Geometry check sheet. Reference: the model listing, model coordinates, mm. Face numbers are marked on the shaded views. A direction names the side the tool comes from. Give positions to 0.01 mm unless a question says otherwise; leave off trailing zeros. Order: outer loops, then holes, each group sorted by start corner. A loop starts at its lowest first (then second) coordinate and runs counter-clockwise, first axis right, second up. Notation, with made-up numbers: M 35.25,16 L 68.25,16 A31 ccw 68.25,52 Z; hole C 51,57 d10. An arc over 180 degrees is marked long. Use CSV: the item, a comma, the result in double quotes. Start each with the question number.
from build123d import *

# Parameters (mm, degrees)
F0_W     = 3.5
F0_H     = 4.8
F1_DEPTH = 19
F3_D     = 5
F3_DEPTH = 10
F3_TIP   = 1.5021515476


with BuildPart() as f1:
    # F0 (on Right) → F1 (new body)
    with BuildSketch(Plane.YZ):
        with Locations((-19.75, 3.4)):
            Rectangle(F0_W, F0_H)
        Polygon((21.5, -1), (21.5, 1), (18, 1), (-18, 1), (-21.5, 1), (-21.5, -1), align=None)
        with Locations((19.75, 3.4)):
            Rectangle(F0_W, F0_H)
    extrude(amount=F1_DEPTH)

    # F3
    with Locations(Plane(origin=(0, 0, -1), x_dir=(1, 0, 0), z_dir=(0, 0, -1))):
        with Locations((9.5, 14), (9.5, -14)):
            Hole(F3_D / 2, depth=F3_DEPTH)
            with Locations((0, 0, -(F3_DEPTH + F3_TIP / 2))):  # 118° drill point
                Cone(0, F3_D / 2, F3_TIP, mode=Mode.SUBTRACT)


solid = f1.part
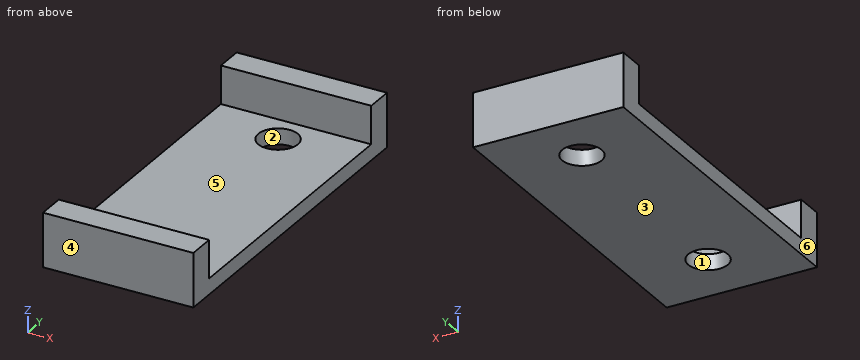
(1) Draft check along Y on the marked faces 1, 2, 3 and 4. Enter one of: +Y half, -Y half, draft (parallel to the pull), parting line (faces both ways), or undercut.
(2) Access from +Z, -Z, +X, -X, +Y, -Y to the whole of each face (thin tool, end or side, straight path). Record for the marked faces 5 and 6.
(3) Thickness scan on line 1 (Y direction, x = 9.5, z = -0.1); line 2 (Y direction, x = 4.5, z = 4.25); line 3 (Y direction, x = 7.5, z = 0). Record the ranges inside material, lowest first.
(4) Sectioned sample at C-C on z = 2.75. Record the cut outline in (x, y), then the cut area to 3 significant figures.
(5) Sectioned sample at B-B on x = 7.5. Record the cut outline in (y, z), then the cut area to 3 significant figures.
(6) Go/stop test with flat-tipped pins: P1, Ø5.5, axis at x = 12.5, y = 5.5, coming from the +Z side; P2, Ø4, axis at x = 9.5, y = -14, coming from the +Z side. Record where each tip stops, or that it passes through.
(7) Sectioned sample at D-D on x = 3.5. Record the cut outline in (y, z).
(8) Sectioned sample at A-A on y = 16. Record the cut outline in (x, z), then the cut area to 3 significant figures.
Responses:
1,face 1,"undercut"
1,face 2,"undercut"
1,face 3,"draft"
1,face 4,"-Y half"
2,face 5,"+Z, +X, -X"
2,face 6,"+Z, -Z, -X, +Y, -Y"
3,line 1,"-21.5 to -16.5, -11.5 to 11.5, 16.5 to 21.5"
3,line 2,"-21.5 to -18, 18 to 21.5"
3,line 3,"-21.5 to -15.5, -12.5 to 12.5, 15.5 to 21.5"
4,outline,"M 0,-21.5 L 19,-21.5 L 19,-18 L 0,-18 Z; M 0,18 L 19,18 L 19,21.5 L 0,21.5 Z"
4,area,"133 mm2"
5,outline,"M -21.5,-1 L -15.5,-1 L -15.5,1 L -18,1 L -18,5.8 L -21.5,5.8 Z; M -12.5,-1 L 12.5,-1 L 12.5,1 L -12.5,1 Z; M 15.5,-1 L 21.5,-1 L 21.5,5.8 L 18,5.8 L 18,1 L 15.5,1 Z"
5,area,"108 mm2"
6,P1,"z = 1"
6,P2,"through"
7,outline,"M -21.5,-1 L 21.5,-1 L 21.5,5.8 L 18,5.8 L 18,1 L -18,1 L -18,5.8 L -21.5,5.8 Z"
8,outline,"M 0,-1 L 8,-1 L 8,1 L 0,1 Z; M 11,-1 L 19,-1 L 19,1 L 11,1 Z"
8,area,"32.0 mm2"
